from build123d import *

# Parameters (mm, degrees)
F0_W     = 50.8
F0_H     = 50.8
F1_DEPTH = 25.4
F2_R     = 8.255
F3_DEPTH = 25.4
F4_DEPTH = 12.7
F5_DEPTH = 12.7
F6_DEPTH = 12.7


with BuildPart() as f1:
    # F0 (on Front) → F1 (new body)
    with BuildSketch(Plane.XZ):
        Rectangle(F0_W, F0_H)
    extrude(amount=F1_DEPTH)

    # F2 (on face) → F3 (cut)
    with BuildSketch(Plane.XZ.offset(25.4)):
        with Locations((-13.0175, 0)):
            Circle(F2_R)
        with BuildLine():
            ThreePointArc((21.2725, 0), (13.0175, 8.255), (4.7625, 0))
            ThreePointArc((4.7625, 0), (13.0175, -8.255), (21.2725, 0))
        make_face()
    extrude(amount=-F3_DEPTH, mode=Mode.SUBTRACT)

    # F4 (cut): a face of the model
    f4_faces = [f1.faces().sort_by_distance(p)[0] for p in [
        (0, -25.4, 0),
    ]]
    extrude(f4_faces, amount=-F4_DEPTH, mode=Mode.SUBTRACT)

    # F5 (cut): a face of the model
    f5_faces = [f1.faces().sort_by_distance(p)[0] for p in [
        (0, -6.35, 25.4),
    ]]
    extrude(f5_faces, amount=-F5_DEPTH, mode=Mode.SUBTRACT)

    # F6 (cut): a face of the model
    f6_faces = [f1.faces().sort_by_distance(p)[0] for p in [
        (0, -6.35, -25.4),
    ]]
    extrude(f6_faces, amount=-F6_DEPTH, mode=Mode.SUBTRACT)


solid = f1.part
Input: part model. Units: mm. Frame: model coordinates. Coordinates: 2 decimals unless noted, no trailing zeros. Loops run counter-clockwise (first coordinate to the right, second up) from the corner with the lowest first, then second, coordinate; pieces in that order, holes last. Notation, with made-up numbers: (9.25, 8) -> (68.25, 8) arc R29 cw to (68.25, 33) -> close; hole circle Ø8 at (19, -32.75). An arc over 180 degrees is marked (long way). Write item = value, one per line. Start each with the question number.
Item 1: Cut plane D-D, the plane z = -3.5. Return loops of the section in (x, y).
Item 2: Cut plane B-B, the plane x = 14.5. Return loops of the section in (y, z), plus the area to 3 significant figures.
Item 3: Material intervals for line 1 (Z direction, x = -13, y = -7.25); line 2 (X direction, y = -11, z = 4.5); line 3 (X direction, y = -10.5, z = 2.75), sorted ascending.
Item 4: Mould query, pull axis Z, two halves, no side actions, for faces 1 (the face through (19.57, -6.44, 5.02)), 2 (the face through (0, -6, 12.7)), 3 (the face through (0, -12.7, 0)). Classes: pulls with the +Z half, pulls with the -Z half, needs draft (parallel to the pull), parting line crosses it, or undercut.
Item 5: Cut plane A-A, the plane z = 0. Return loops of the section in (x, y).
Item 6: Cut plane C-C, the plane y = -9.25. Return loops of the section in (x, z) (1 decimal), plus the area to 3 significant figures.
Ans:
q1.outline = (-25.4, -12.7) -> (-20.49, -12.7) -> (-20.49, 0) -> (-25.4, 0) -> close; (-5.54, -12.7) -> (5.54, -12.7) -> (5.54, 0) -> (-5.54, 0) -> close; (20.49, -12.7) -> (25.4, -12.7) -> (25.4, 0) -> (20.49, 0) -> close
q2.outline = (-12.7, -12.7) -> (0, -12.7) -> (0, -8.12) -> (-12.7, -8.12) -> close; (-12.7, 8.12) -> (0, 8.12) -> (0, 12.7) -> (-12.7, 12.7) -> close
q2.area = 116 mm²
q3.line_1 = -12.7 to -8.25, 8.25 to 12.7
q3.line_2 = -25.4 to -19.94, -6.1 to 6.1, 19.94 to 25.4
q3.line_3 = -25.4 to -20.8, -5.23 to 5.23, 20.8 to 25.4
q4.face_1 = undercut
q4.face_2 = pulls with the +Z half
q4.face_3 = needs draft
q5.outline = (-25.4, -12.7) -> (-21.27, -12.7) -> (-21.27, 0) -> (-25.4, 0) -> close; (-4.76, -12.7) -> (4.76, -12.7) -> (4.76, 0) -> (-4.76, 0) -> close; (21.27, -12.7) -> (25.4, -12.7) -> (25.4, 0) -> (21.27, 0) -> close
q6.outline = (-25.4, -12.7) -> (25.4, -12.7) -> (25.4, 12.7) -> (-25.4, 12.7) -> close; hole circle Ø16.5 at (-13, 0); hole circle Ø16.5 at (13, 0)
q6.area = 862 mm²
